from build123d import *

# Parameters (mm, degrees)
SKETCH2_W           = 19.05
SKETCH2_H           = 83.058
BOSS_EXTRUDE1_DEPTH = 3.175
FILLET1_R           = 10.16
SKETCH3_R           = 1.5875
CUT_EXTRUDE1_DEPTH  = 3.175


with BuildPart() as part:
    # Sketch2 → Boss-Extrude1 (new body)
    with BuildSketch(Plane.XY):
        with Locations((-9.525, 41.529)):
            Rectangle(SKETCH2_W, SKETCH2_H)
    extrude(amount=BOSS_EXTRUDE1_DEPTH)

    # Fillet1
    # the kernel refuses this fillet: 10.16 mm, written as the material it takes off along each edge
    with BuildSketch(Plane(origin=(-19.05, 0, -25.4), x_dir=(1, 0, 0), z_dir=(0, 0, 1)), Plane(origin=(-19.05, 83.058, -25.4), x_dir=(0, -1, 0), z_dir=(0, 0, 1)), Plane(origin=(0, 83.058, -25.4), x_dir=(-1, 0, 0), z_dir=(0, 0, 1))) as fillet1_piece_1:
        with BuildLine():
            CenterArc((FILLET1_R, FILLET1_R), FILLET1_R, 180, 90)
            Line((0, FILLET1_R), (0, 0))
            Line((0, 0), (FILLET1_R, 0))
        make_face()
    extrude(amount=53.975, mode=Mode.SUBTRACT)
    with BuildSketch(Plane(origin=(0, 0, -25.4), x_dir=(-1, 0, 0), z_dir=(0, 0, 1))) as fillet1_piece_2:
        with BuildLine():
            CenterArc((FILLET1_R, -FILLET1_R), FILLET1_R, 90, 90)
            Line((0, -FILLET1_R), (0, 0))
            Line((0, 0), (FILLET1_R, 0))
        make_face()
    extrude(amount=53.975, mode=Mode.SUBTRACT)

    # Sketch3 → Cut-Extrude1 (cut)
    with BuildSketch(Plane.XY.offset(3.175)):
        with Locations((-9.525, 12.719863167)):
            Circle(SKETCH3_R)
        with Locations((-9.525, 70.338136833)):
            Circle(SKETCH3_R)
    extrude(amount=-CUT_EXTRUDE1_DEPTH, mode=Mode.SUBTRACT)


solid = part.part
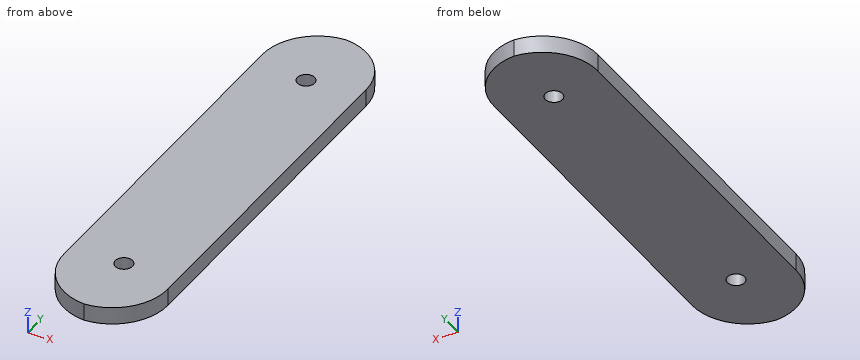
Here's how the part is built. I have some questions about the finished solid (model axes, mm). Give positions to 0.01 mm unless a question says otherwise; leave off trailing zeros. Order: outer loops, then holes, each group sorted by start corner. A loop starts at its lowest first (then second) coordinate and runs counter-clockwise, first axis right, second up. Notation, with made-up numbers: (-12, 53) -> (11, 53) arc R29 cw to (11, 76) -> close; hole circle Ø4 at (-17, 50). An arc over 180 degrees is marked (long way). Use a Markdown table: item, result. Add a question column.
Item 1: Imagine slicing it at A-A on z = 0.55. Give the number of separate pieces and of enclosed holes in the cut face, plus the area to 3 significant figures.
Item 2: Imagine slicing it at B-B on y = 12. Please give me the cut outline in (x, z) (3 decimals), plus the area to 3 significant figures.
Item 3: I need wall thicknesses on line 1 (Y direction, x = -9.5, z = 2.7); line 2 (Y direction, x = -9, z = 0.85); line 3 (X direction, y = 11.5, z = 0.7). Which ranges of each line are inside material? Lowest first, please.
Item 4: Imagine slicing it at C-C on x = -16.25. Please give me the cut outline in (y, z) (3 decimals), plus the area to 3 significant figures.
Item 5: Will these pins go through, and if not, where does the flat tip stop? pin 1 (3 mm diameter, centred on x = -9.52, y = 12.72, fed in from -Z); pin 2 (1 mm diameter, centred on x = -6, z = 0.5, fed in from -Y); pin 3 (1.5 mm diameter, centred on x = -16, z = 1.5, fed in from -Y).
Data:
| question | item | result |
|---|---|---|
| 1 | separate pieces | 1 |
| 1 | enclosed holes | 2 |
| 1 | area | 1,480 mm² |
| 2 | outline | (-19.05, 0) -> (-10.94, 0) -> (-10.94, 3.175) -> (-19.05, 3.175) -> close; (-8.11, 0) -> (0, 0) -> (0, 3.175) -> (-8.11, 3.175) -> close |
| 2 | area | 51.5 mm² |
| 3 | line 1 | y = 0.02 to 11.13, 14.31 to 68.75, 71.93 to 83.04 |
| 3 | line 2 | y = 0.07 to 11.22, 14.22 to 68.84, 71.84 to 82.99 |
| 3 | line 3 | x = -19.05 to -10.54, -8.51 to 0 |
| 4 | outline | (3.156, 0) -> (79.902, 0) -> (79.902, 3.175) -> (3.156, 3.175) -> close |
| 4 | area | 244 mm² |
| 5 | pin 1 | passes through |
| 5 | pin 2 | stops at y = 0.68 |
| 5 | pin 3 | stops at y = 2.24 |
